Job drawing, mm, ordinate dimensions from the low corner. One solid piece. A direction names the side the tool comes from. Round coordinates to 2 decimals unless told otherwise and drop trailing zeros. Order: outer loops, then holes, each group sorted by start corner. A loop starts at its lowest first (then second) coordinate and runs counter-clockwise, first axis right, second up. Notation, with made-up numbers: (45.25, -15) -> (89.25, -15) arc R24 ccw to (89.25, 8) -> close; hole circle Ø7 at (27.5, 4.25). An arc over 180 degrees is marked (long way). Return JSON: item names as keys, results as strings. Group by question number.
Q1. Cut at A-A (y = 131.5). Write the cut outline in (x, z), then the cut area to 3 significant figures.
Q2. Probe line 1 along X through (y, z) = (132.5, 14); line 2 along Y through (x, z) = (26.5, 30.5); line 3 along X through (y, z) = (17, 29). List the from-to ranges inside material, lowest first.
Q3. Cut at C-C (y = 61.5). Write the cut outline in (x, z), then the cut area to 3 significant figures.
Q4. Flat gauge pins, fed straight in: pin 1 (15 mm diameter, centred on x = 156.5, z = 14.5, fed in from -Y); pin 2 (1 mm diameter, centred on y = 83, z = 5.5, fed in from -X); pin 3 (17.5 mm diameter, centred on x = 160, z = 20, fed in from -Y). Where does each tip first touch, or does it go through?
Q5. Cut at D-D (z = 36). Write the cut outline in (x, y).
Q6. Cut at B-B (x = 20). Write the cut outline in (y, z), then the cut area to 3 significant figures.
Q7. Mould opens along Y. For the marked faces 1, 2 and 3 say: +Y half, -Y half, draft (parallel to the pull), parting line (faces both ways), or undercut.
Q8. Which spindle directions (+Z, -Z, +X, -X, +Y, -Y) get a long thin tool onto all of the face, cutting with end or side? Do the marked faces 4, 5 and 6. Say none if no direction does.
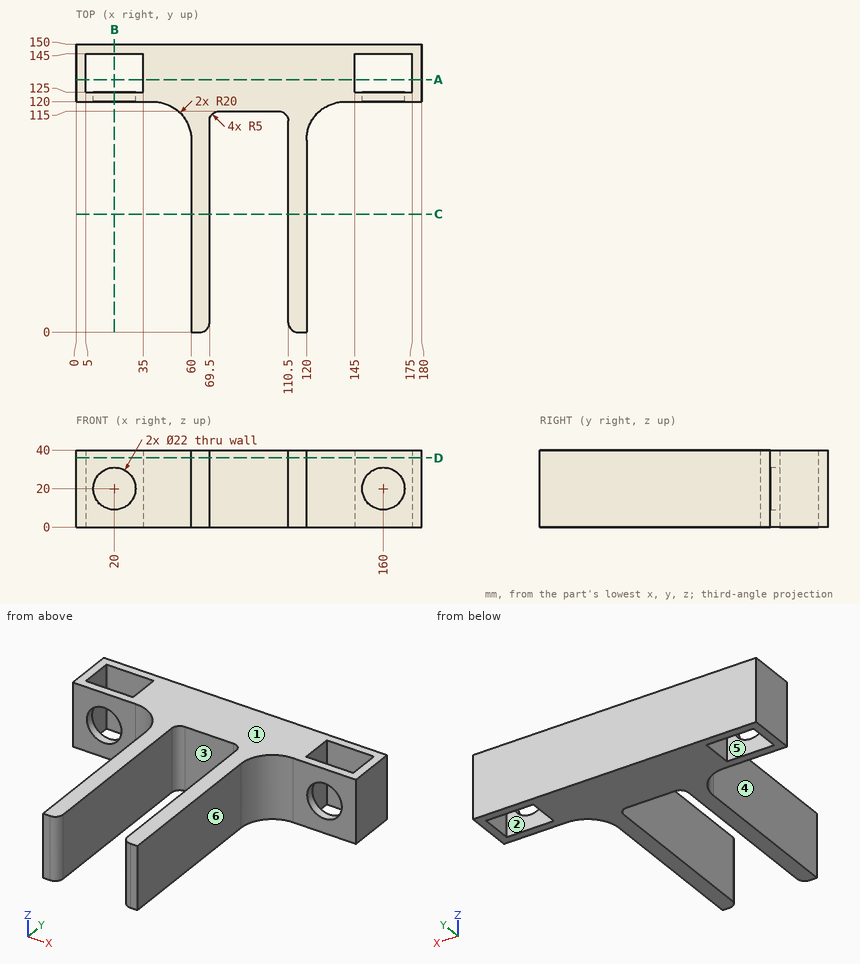
Solution:
{
 "1": {"outline": "(0, 0) -> (5, 0) -> (5, 40) -> (0, 40) -> close; (35, 0) -> (145, 0) -> (145, 40) -> (35, 40) -> close; (175, 0) -> (180, 0) -> (180, 40) -> (175, 40) -> close", "area": "4,800 mm²"},
 "2": {"line 1": "x = 0 to 5, 35 to 145, 175 to 180", "line 2": "y = 120 to 125, 145 to 150", "line 3": "x = 60 to 69.5, 110.5 to 120"},
 "3": {"outline": "(60, 0) -> (69.5, 0) -> (69.5, 40) -> (60, 40) -> close; (110.5, 0) -> (120, 0) -> (120, 40) -> (110.5, 40) -> close", "area": "760 mm²"},
 "4": {"pin 1": "stops at y = 120", "pin 2": "stops at x = 60", "pin 3": "stops at y = 145"},
 "5": {"outline": "(0, 120) -> (40, 120) arc R20 cw to (60, 100) -> (60, 0) -> (64.5, 0) arc R5 ccw to (69.5, 5) -> (69.5, 110) arc R5 cw to (74.5, 115) -> (105.5, 115) arc R5 cw to (110.5, 110) -> (110.5, 5) arc R5 ccw to (115.5, 0) -> (120, 0) -> (120, 100) arc R20 cw to (140, 120) -> (180, 120) -> (180, 150) -> (0, 150) -> close; hole (5, 125) -> (35, 125) -> (35, 145) -> (5, 145) -> close; hole (145, 125) -> (175, 125) -> (175, 145) -> (145, 145) -> close"},
 "6": {"outline": "(120, 0) -> (125, 0) -> (125, 9) -> (120, 9) -> close; (120, 31) -> (125, 31) -> (125, 40) -> (120, 40) -> close; (145, 0) -> (150, 0) -> (150, 40) -> (145, 40) -> close", "area": "290 mm²"},
 "7": {"face 1": "draft", "face 2": "undercut", "face 3": "-Y half"},
 "8": {"face 4": "+Z, -Z, -X, -Y", "face 5": "+Z, -Z", "face 6": "+Z, -Z, +X, -Y"}
}
